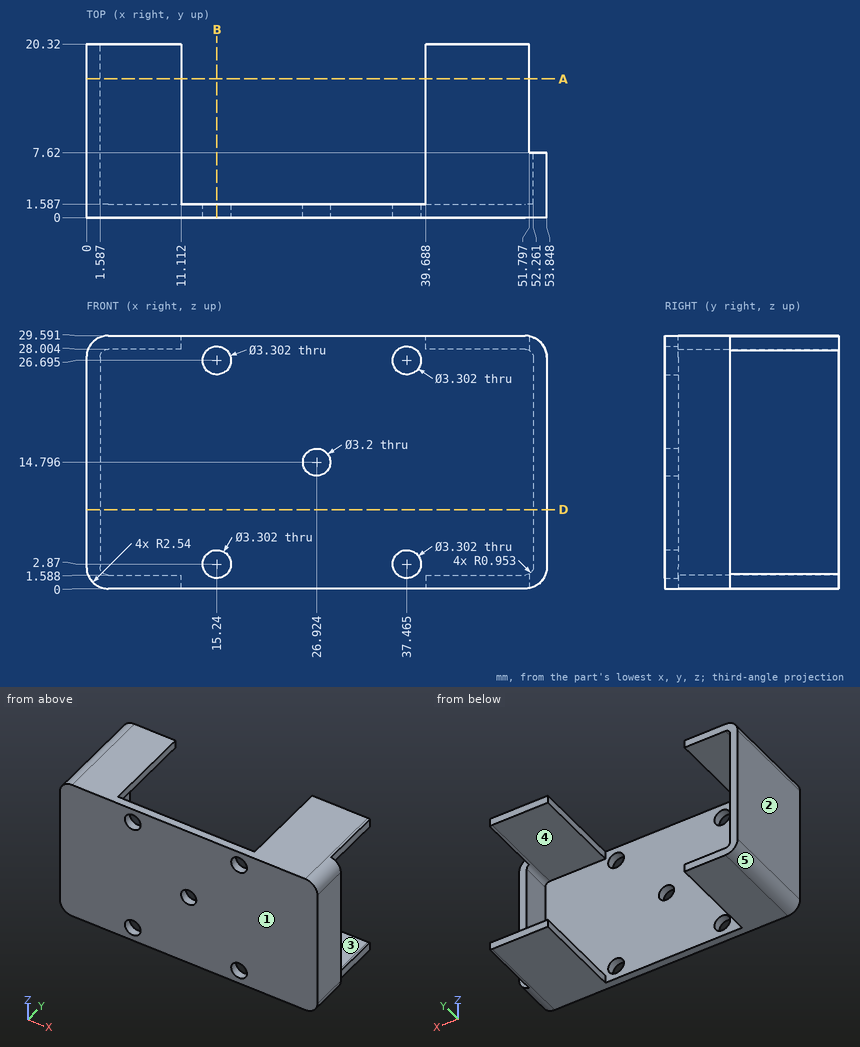
Part print with two shaded views. Sizes in mm from the minimum x, y, z corner. A direction names the side the tool comes from. Round coordinates to 2 decimals unless told otherwise and drop trailing zeros. Loops run counter-clockwise (first coordinate to the right, second up) from the corner with the lowest first, then second, coordinate; pieces in that order, holes last. Notation, with made-up numbers: M 36.5,16.25 L 50.5,16.25 A3 ccw 50.5,20.25 Z; hole C 30.5,-11 d1. An arc over 180 degrees is marked long. Put each result on its own line as item: value. Start each with the question number.
Item 1: 3-axis set-ups, long thin cutter, end or side, ignore diameter. For the marked faces 4 and 5: which of +Z, -Z, +X, -X, +Y, -Y reach the whole face in a straight line?
Item 2: Drop flat-ended pins along their axis: P1, Ø2.5, axis at x = 53.5, z = 11, coming from the +Y side; P2, Ø0.8, axis at y = 15, z = 29, coming from the +X side; P3, Ø4.5, axis at x = 37.47, z = 2.87, coming from the +Y side; P4, Ø10, axis at x = 31.5, y = 9.5, coming from the +Z side. Give the stop position or say it passes through.
Item 3: Drill centre lines: line 1 along Z through (x, y) = (15.24, 1.3) (1 decimal); line 2 along Z through (x, y) = (47, 5.25); line 3 along X through (y, z) = (3.5, 12). Where is each one in solid material? Low to high.
Item 4: Cut at B-B (x = 15.24). List the corners of the cut face in (y, z) (1 decimal).
Item 5: Mould opens along X. For the marked faces 1, 2 and 3 say: released by +X, released by -X, zero draft, split by the parting line, or undercut.
Item 6: Cut at A-A (y = 16.25). Give the number of separate pieces and of enclosed holes in the cut face, then the cut area to 3 significant figures.
Item 7: Cut at D-D (z = 9.25). List the corners of the cut face in (x, y), then the cut area to 3 significant figures.
Answer block:
1. face 4: +Y
1. face 5: -Z, -X, +Y, -Y
2. P1: y = 7.62
2. P2: x = 51.8
2. P3: y = 1.59
2. P4: through
3. line 1: 0 to 1.2, 4.5 to 25, 28.3 to 29.6
3. line 2: 0 to 1.59, 28 to 29.59
3. line 3: 0 to 1.59, 52.26 to 53.85
4. outline: M 0,0 L 1.6,0 L 1.6,1.2 L 0,1.2 Z; M 0,4.5 L 1.6,4.5 L 1.6,25 L 0,25 Z; M 0,28.3 L 1.6,28.3 L 1.6,29.6 L 0,29.6 Z
5. face 1: zero draft
5. face 2: released by -X
5. face 3: undercut
6. separate pieces: 3
6. enclosed holes: 0
6. area: 113 mm2
7. outline: M 0,0 L 53.85,0 L 53.85,7.62 L 52.26,7.62 L 52.26,1.59 L 1.59,1.59 L 1.59,20.32 L 0,20.32 Z
7. area: 125 mm2
